Geometry check sheet. Reference: the model listing, model coordinates, mm. A direction names the side the tool comes from. Give positions to 0.01 mm unless a question says otherwise; leave off trailing zeros. Loops run counter-clockwise (first coordinate to the right, second up) from the corner with the lowest first, then second, coordinate; pieces in that order, holes last. Notation, with made-up numbers: (5, 66) -> (56, 66) arc R27 ccw to (56, 102) -> close; hole circle Ø9 at (80.5, 57). An arc over 180 degrees is marked (long way). Answer in a Markdown table with one row per item. Add a question column.
```python
from build123d import *

# Parameters (mm, degrees)
CHANFREIN1_SIZE = 0.6


with BuildPart() as part:
    # Esquisse1 → Base-Révolution (revolve)
    with BuildSketch(Plane.XY, mode=Mode.PRIVATE) as base_r_volution_sk:
        Polygon((0, 0), (0, 7), (2, 7), (2, 5), (10, 5), (10, 4), (24, 4), (24, 3.3), (25, 3.3), (25, 4), (34, 4), (34, 0), align=None)
    revolve(base_r_volution_sk.sketch.rotate(Axis((-12.574722565, 0, 0), (1, 0, 0)), 90), axis=Axis((-12.574722565, 0, 0), (1, 0, 0)))

    # Chanfrein1
    chanfrein1_edges = [part.edges().sort_by_distance(p)[0] for p in [
        (34, 0, -4),
    ]]
    chamfer(chanfrein1_edges, length=CHANFREIN1_SIZE)


solid = part.part
```
1. Sectioned sample at A-A (y = 0). Enter the section's corners in (x, z), plus the area to 3 significant figures.
2. Access from +Z, -Z, +X, -X, +Y, -Y to the whole of each face (thin tool, end or side, straight path). Record for faces 1 (the face through (1.01, 6.21, 3.23)), 2 (the face through (24.51, -2.23, -2.43)), 3 (the face through (6, 0, -5)).
3. Sectioned sample at C-C (x = 17). Enter the section's corners in (y, z).
4. Release check for a two-part mould opening along X. For faces 4 (the face through (17.098, 3.905, -0.867)), 5 (the face through (25, -3, 2)), 6 (the face through (2, -5, -2)) record: released by +X, released by -X, zero draft, split by the parting line, or undercut.
5. Sectioned sample at D-D (y = -5.5). Enter the section's corners in (x, z), plus the area to 3 significant figures.
6. Material ranges on L1, parallel to Y at x = 3.5, z = 0.25; L2, parallel to Y at x = 27.5, z = 0; L3, parallel to X at y = -1, z = -5, recorded low to high. Write a range as from..to.
7. Gauge pin test, flat ends, axial feed: pin 1 Ø6 at (x, z) = (8, 4.5) entering from -Y; pin 2 Ø4 at (y, z) = (0, -3) entering from -X; pin 3 Ø4 at (x, y) = (11.5, 1.5) entering from +Z; pin 4 Ø1.5 at (x, z) = (30.5, -5.5) entering from -Y. Record the tip position at first contact, or that the pin passes through.
Response:
| question | item | result |
|---|---|---|
| 1 | outline | (0, -7) -> (2, -7) -> (2, -5) -> (10, -5) -> (10, -4) -> (24, -4) -> (24, -3.3) -> (25, -3.3) -> (25, -4) -> (33.4, -4) -> (34, -3.4) -> (34, 3.4) -> (33.4, 4) -> (25, 4) -> (25, 3.3) -> (24, 3.3) -> (24, 4) -> (10, 4) -> (10, 5) -> (2, 5) -> (2, 7) -> (0, 7) -> close |
| 1 | area | 298 mm2 |
| 2 | face 1 | +X, -X |
| 2 | face 2 | none |
| 2 | face 3 | +X |
| 3 | outline | circle Ø8 at (0, 0) |
| 4 | face 4 | zero draft |
| 4 | face 5 | undercut |
| 4 | face 6 | released by +X |
| 5 | outline | (0, -4.33) -> (2, -4.33) -> (2, 4.33) -> (0, 4.33) -> close |
| 5 | area | 17.3 mm2 |
| 6 | L1 | y = -4.99..4.99 |
| 6 | L2 | y = -4..4 |
| 6 | L3 | x = 0..2 |
| 7 | pin 1 | stops at y = -4.77 |
| 7 | pin 2 | stops at x = 0 |
| 7 | pin 3 | stops at z = 5 |
| 7 | pin 4 | passes through |
